Verification items for the finished model (mm, model axes). A direction names the side the tool comes from. Coordinates: 2 decimals unless noted, no trailing zeros. Loops run counter-clockwise (first coordinate to the right, second up) from the corner with the lowest first, then second, coordinate; pieces in that order, holes last. Notation, with made-up numbers: (-38.5, 52.25) -> (-22.5, 52.25) arc R23 ccw to (-22.5, 89.25) -> close; hole circle Ø9 at (74, 62.5). An arc over 180 degrees is marked (long way). Write item = value, one per line.
```python
from build123d import *

# Parameters (mm, degrees)
SKETCH1_W                      = 304.8
SKETCH1_H                      = 76.2
BASE_FLANGE1_DEPTH             = 3.03784
EDGE_FLANGE1_STRIP_W           = 18.50136
EDGE_FLANGE1_STRIP_H           = 3.03784
EDGE_FLANGE1_STRIP_CUT_DEPTH   = 76.2
EDGE_FLANGE1_STRIP_2_W         = 18.50136
EDGE_FLANGE1_STRIP_2_H         = 3.03784
EDGE_FLANGE1_STRIP_CUT_2_DEPTH = 76.2
EDGE_FLANGE1_DEPTH             = 76.2
EDGE_FLANGE1_BEND_DEPTH        = 76.2
EDGE_FLANGE2_DEPTH             = 292.37432
EDGE_FLANGE2_BEND_DEPTH        = 292.37432
F_3_8_CLEARANCE_HOLE1_D        = 10.31748
F_11_0_191_DIAMETER_HOLE1_D    = 4.8514
FILLET1_R                      = 6.35


# Sheet-metal steps are written as plain solids
with BuildPart() as part:
    # Sketch1 → Base-Flange1 (new body)
    with BuildSketch(Plane(origin=(0, 0, 0), x_dir=(1, 0, 0), z_dir=(0, 1, 0))):
        with Locations((152.4, 38.1)):
            Rectangle(SKETCH1_W, SKETCH1_H)
    extrude(amount=-BASE_FLANGE1_DEPTH)

    # Edge-Flange1 strip (across the edge) → Edge-Flange1 strip cut (cut)
    with BuildSketch(Plane.XY.offset(-76.2)):
        with Locations((-3.03784, -1.51892)):
            Rectangle(EDGE_FLANGE1_STRIP_W, EDGE_FLANGE1_STRIP_H)
    extrude(amount=EDGE_FLANGE1_STRIP_CUT_DEPTH, mode=Mode.SUBTRACT)

    # Edge-Flange1 strip 2 (across the edge) → Edge-Flange1 strip cut 2 (cut)
    with BuildSketch(Plane(origin=(304.8, 0, 0), x_dir=(-1, 0, 0), z_dir=(0, 0, -1))):
        with Locations((-3.03784, -1.51892)):
            Rectangle(EDGE_FLANGE1_STRIP_2_W, EDGE_FLANGE1_STRIP_2_H)
    extrude(amount=EDGE_FLANGE1_STRIP_CUT_2_DEPTH, mode=Mode.SUBTRACT)

    # Edge-Flange1 section (across the edge) → Edge-Flange1 (add)
    with BuildSketch(Plane.XY.offset(-76.2)):
        with BuildLine():
            Line((0, 3.175), (0, 35.06216))
            Line((0, 35.06216), (3.03784, 35.06216))
            Line((3.03784, 35.06216), (3.03784, 3.175))
            ThreePointArc((3.03784, 3.175), (3.96777597, 0.92993597), (6.21284, 0))
            Line((6.21284, 0), (6.21284, -3.03784))
            ThreePointArc((6.21284, -3.03784), (1.819698706, -1.218141294), (0, 3.175))
        make_face()
    extrude(amount=EDGE_FLANGE1_DEPTH)

    # Edge-Flange1 section 2 (across the edge) → Edge-Flange1 bend (add)
    with BuildSketch(Plane(origin=(304.8, 0, 0), x_dir=(-1, 0, 0), z_dir=(0, 0, -1))):
        with BuildLine():
            Line((0, 3.175), (0, 35.06216))
            Line((0, 35.06216), (3.03784, 35.06216))
            Line((3.03784, 35.06216), (3.03784, 3.175))
            ThreePointArc((3.03784, 3.175), (3.96777597, 0.92993597), (6.21284, 0))
            Line((6.21284, 0), (6.21284, -3.03784))
            ThreePointArc((6.21284, -3.03784), (1.819698706, -1.218141294), (0, 3.175))
        make_face()
    extrude(amount=EDGE_FLANGE1_BEND_DEPTH)

    # Edge-Flange2 section (across the edge) → Edge-Flange2 (add)
    with BuildSketch(Plane(origin=(6.21284, 0, 3.175), x_dir=(0, 0, -1), z_dir=(1, 0, 0))):
        with BuildLine():
            Line((-3.03784, 3.175), (-3.03784, 28.71216))
            Line((-3.03784, 28.71216), (0, 28.71216))
            Line((0, 28.71216), (0, 3.175))
            ThreePointArc((0, 3.175), (0.92993597, 0.92993597), (3.175, 0))
            Line((3.175, 0), (3.175, -3.03784))
            ThreePointArc((3.175, -3.03784), (-1.218141294, -1.218141294), (-3.03784, 3.175))
        make_face()
    extrude(amount=EDGE_FLANGE2_DEPTH)

    # Edge-Flange2 section 2 (across the edge) → Edge-Flange2 bend (add)
    with BuildSketch(Plane(origin=(298.58716, 0, -79.375), x_dir=(0, 0, 1), z_dir=(-1, 0, 0))):
        with BuildLine():
            Line((-3.03784, 3.175), (-3.03784, 28.71216))
            Line((-3.03784, 28.71216), (0, 28.71216))
            Line((0, 28.71216), (0, 3.175))
            ThreePointArc((0, 3.175), (0.92993597, 0.92993597), (3.175, 0))
            Line((3.175, 0), (3.175, -3.03784))
            ThreePointArc((3.175, -3.03784), (-1.218141294, -1.218141294), (-3.03784, 3.175))
        make_face()
    extrude(amount=EDGE_FLANGE2_BEND_DEPTH)

    # 3/8 Clearance Hole1 (through all)
    with Locations(Plane(origin=(0, -3.03784, 0), x_dir=(-1, 0, 0), z_dir=(0, -1, 0))):
        with Locations((-88.9, 38.1), (-215.9, 38.1)):
            Hole(F_3_8_CLEARANCE_HOLE1_D / 2)

    # #11 (0.191) Diameter Hole1 (through all)
    with Locations(Plane(origin=(304.8, 0, 0), x_dir=(0, 0, -1), z_dir=(1, 0, 0))):
        with Locations((12.7, 15.6337), (38.1, 15.6337), (63.5, 15.6337)):
            Hole(F_11_0_191_DIAMETER_HOLE1_D / 2)

    # Fillet1
    fillet1_edges = [part.edges().sort_by_distance(p)[0] for p in [
        (1.51892, 35.06216, 0),
        (6.21284, 28.71216, 4.69392),
        (1.51892, 35.06216, -76.2),
        (298.58716, 28.71216, 4.69392),
        (6.21284, 28.71216, -80.89392),
        (303.28108, 35.06216, 0),
        (298.58716, 28.71216, -80.89392),
        (303.28108, 35.06216, -76.2),
    ]]
    fillet(fillet1_edges, radius=FILLET1_R)


solid = part.part
```
1) Material ranges on line 1 (Z direction, x = 58, y = 12) (3 decimals); line 2 (X direction, y = 19, z = -66); line 3 (Y direction, x = 170, z = -62), recorded low to high.
Ans:
line_1 = -82.413 to -79.375, 3.175 to 6.213
line_2 = 0 to 3.04, 301.76 to 304.8
line_3 = -3.04 to 0
2) Release check for a two-part mould opening along X. For faces 1 (the face through (301.762, 19, -38)), 2 (the face through (210.746, -1.498, -38.327)), 3 (the face through (6.213, 10, 4)), 4 (the face through (296.78, 26.8, 4.67)) record: pulls with the +X half, pulls with the -X half, needs draft (parallel to the pull), parting line crosses it, or undercut.
Ans:
face_1 = undercut
face_2 = undercut
face_3 = pulls with the -X half
face_4 = pulls with the +X half
3) Sectioned sample at C-C, the plane x = 103. Record the cut outline in (y, z) (3 decimals).
Ans:
outline = (-3.038, -76.2) arc R6.213 ccw to (3.175, -82.413) -> (28.712, -82.413) -> (28.712, -79.375) -> (3.175, -79.375) arc R3.175 cw to (0, -76.2) -> (0, 0) arc R3.175 cw to (3.175, 3.175) -> (28.712, 3.175) -> (28.712, 6.213) -> (3.175, 6.213) arc R6.213 ccw to (-3.038, 0) -> close
4) Sectioned sample at B-B, the plane y = 32. Record the cut outline in (x, z), plus the area to 3 significant figures.
Ans:
outline = (0, -75.28) -> (3.04, -75.28) -> (3.04, -0.92) -> (0, -0.92) -> close; (301.76, -75.28) -> (304.8, -75.28) -> (304.8, -0.92) -> (301.76, -0.92) -> close
area = 452 mm2
5) Sectioned sample at A-A, the plane x = 215.9. Record the cut outline in (y, z) (3 decimals), plus the area to 3 significant figures.
Ans:
outline = (-3.038, -76.2) arc R6.213 ccw to (3.175, -82.413) -> (28.712, -82.413) -> (28.712, -79.375) -> (3.175, -79.375) arc R3.175 cw to (0, -76.2) -> (0, -43.259) -> (-3.038, -43.259) -> close; (-3.038, -32.941) -> (0, -32.941) -> (0, 0) arc R3.175 cw to (3.175, 3.175) -> (28.712, 3.175) -> (28.712, 6.213) -> (3.175, 6.213) arc R6.213 ccw to (-3.038, 0) -> close
area = 400 mm2
6) Tool access check on faces 5 (the face through (303.26, 18.04, -63.82)), 6 (the face through (298.587, 10, -81)), 7 (the face through (3.038, 19, -39)), 8 (the face through (298.587, 10, 4)), 9 (the face through (150, 0, -39)). Record the directions out of +Z, -Z, +X, -X, +Y, -Y that give a thin tool (end or side, any length) a straight path to the whole face; none if there is none.
Ans:
face_5 = +X, -X
face_6 = -Z, +X, +Y, -Y
face_7 = +Z, -Z, +Y
face_8 = +Z, +X, +Y, -Y
face_9 = +Y
7) Depth check by flat-ended pin: pin 1 Ø0.9 at (x, z) = (106.5, -81.5) entering from +Y; pin 2 Ø7 at (x, y) = (303, 13.5) entering from -Z; pin 3 Ø1.9 at (y, z) = (6.5, -79.5) entering from -X; pin 4 Ø3 at (y, z) = (15.63, -12.7) entering from -X. Enter the tip coordinate at first touch or a pass-through.
Ans:
pin_1 = 28.71
pin_2 = -76.2
pin_3 = 6.21
pin_4 = through
